```python
from build123d import *

# Parameters (mm, degrees)
SKETCH1_R           = 6.5
BOSS_EXTRUDE1_DEPTH = 25
EXTRUDE_THIN1_START = 0.5
SKETCH1_4_R         = 3.5
SKETCH1_4_R_2       = 3
EXTRUDE_THIN1_DEPTH = 20
BOSS_EXTRUDE2_START = 0.8
SKETCH1_5_R         = 5.5
SKETCH1_5_R_2       = 3
BOSS_EXTRUDE2_DEPTH = 19.5
BOSS_EXTRUDE3_START = 0.3
SKETCH1_6_R         = 6.5
SKETCH1_6_R_2       = 5.5
BOSS_EXTRUDE3_DEPTH = 21
BOSS_EXTRUDE4_START = 1
BOSS_EXTRUDE4_DEPTH = 1
FILLET1_R           = 0.5


with BuildPart() as part:
    # Sketch1 → Boss-Extrude1 (new body)
    with BuildSketch(Plane(origin=(0, 0, 0), x_dir=(0, 0, -1), z_dir=(1, 0, 0))):
        Polygon((-15, -3), (-13.5, -1.5), (-13.5, 6), (-6.5, 6), (-5, 9), (5, 9), (6.5, 6), (13.5, 6), (13.5, -1.5), (15, -3), (15, -9), (5, -9), (3.5, -7.5), (-3.5, -7.5), (-5, -9), (-15, -9), align=None)
        Circle(SKETCH1_R, mode=Mode.SUBTRACT)
    extrude(amount=BOSS_EXTRUDE1_DEPTH)



with BuildPart() as body_2:
    # Sketch1_4 → Extrude-Thin1 (new body)
    with BuildSketch(Plane(origin=(0, 0, 0), x_dir=(0, 0, -1), z_dir=(1, 0, 0)).offset(EXTRUDE_THIN1_START)):
        Circle(SKETCH1_4_R)
        Circle(SKETCH1_4_R_2, mode=Mode.SUBTRACT)
    extrude(amount=EXTRUDE_THIN1_DEPTH)

    # Sketch1_5 → Boss-Extrude2 (add)
    with BuildSketch(Plane(origin=(0, 0, 0), x_dir=(0, 0, -1), z_dir=(1, 0, 0)).offset(BOSS_EXTRUDE2_START)):
        Circle(SKETCH1_5_R)
        Circle(SKETCH1_5_R_2, mode=Mode.SUBTRACT)
    extrude(amount=BOSS_EXTRUDE2_DEPTH)


with BuildPart() as part_1:
    add(part.part)

    add(body_2.part)  # Boss-Extrude3 merges body 2
    # Sketch1_6 → Boss-Extrude3 (add)
    with BuildSketch(Plane(origin=(0, 0, 0), x_dir=(0, 0, -1), z_dir=(1, 0, 0)).offset(BOSS_EXTRUDE3_START)):
        Circle(SKETCH1_6_R)
        with Locations(Location((0, 0, 0), (0, 0, 180))):
            Circle(SKETCH1_6_R_2, mode=Mode.SUBTRACT)
    extrude(amount=BOSS_EXTRUDE3_DEPTH)

    # Sketch3 → Boss-Extrude4 (add)
    with BuildSketch(Plane(origin=(21.3, 0, 0), x_dir=(0, 0, -1), z_dir=(1, 0, 0)).offset(BOSS_EXTRUDE4_START)):
        with BuildLine():
            Line((-1.039258499, -5.400920456), (-1.22821459, -6.382905993))
            ThreePointArc((-1.22821459, -6.382905993), (0, 6.5), (1.22821459, -6.382905993))
            Line((1.22821459, -6.382905993), (1.039258499, -5.400920456))
            ThreePointArc((1.039258499, -5.400920456), (1.377808725, -4.340610122), (2.487175706, -4.250171409))
            ThreePointArc((2.487175706, -4.250171409), (3.080776399, -4.371188169), (3.635318393, -4.12728242))
            ThreePointArc((3.635318393, -4.12728242), (0, 5.5), (-3.635318393, -4.12728242))
            ThreePointArc((-3.635318393, -4.12728242), (-3.080776399, -4.371188169), (-2.487175706, -4.250171409))
            ThreePointArc((-2.487175706, -4.250171409), (-1.377808725, -4.340610122), (-1.039258499, -5.400920456))
        make_face()
    extrude(amount=BOSS_EXTRUDE4_DEPTH)

    # Fillet1
    fillet1_edges = [part_1.edges().sort_by_distance(p)[0] for p in [
        (25, -2.25, 14.25),
        (25, -6, 15),
        (0, 2.25, 13.5),
        (0, 6, 10),
        (0, 7.5, 5.75),
        (0, 9, 0),
        (0, 7.5, -5.75),
        (0, 6, -10),
        (0, 2.25, -13.5),
        (0, -2.25, -14.25),
        (0, -6, -15),
        (0, -6, 15),
        (0, -2.25, 14.25),
        (12.5, -1.5, 13.5),
        (12.5, 6, 13.5),
        (12.5, 6, 6.5),
        (12.5, 9, 5),
        (12.5, 9, -5),
        (12.5, 6, -6.5),
        (12.5, 6, -13.5),
        (12.5, -1.5, -13.5),
        (12.5, -3, -15),
        (12.5, -3, 15),
        (25, -6, -15),
        (25, -2.25, -14.25),
        (25, 2.25, -13.5),
        (25, 6, -10),
        (25, 7.5, -5.75),
        (25, 9, 0),
        (25, 7.5, 5.75),
        (25, 6, 10),
        (25, 2.25, 13.5),
    ]]
    fillet(fillet1_edges, radius=FILLET1_R)


solid = part_1.part
```
Input: part model. Units: mm. Frame: model coordinates. A direction names the side the tool comes from. Round coordinates to 2 decimals unless told otherwise and drop trailing zeros. Order: outer loops, then holes, each group sorted by start corner. A loop starts at its lowest first (then second) coordinate and runs counter-clockwise, first axis right, second up. Notation, with made-up numbers: (64, 62) - (119, 62) arc R10 ccw to (119, 79) - close; hole circle Ø3 at (-29, 62). An arc over 180 degrees is marked (long way). One line per question, with ' | ' between items. Start each with the question number.
1) Set-up query: faces 1 (the flat face through (12, -7.5, 0)), 2 (the flat face through (12, 2, 13.5)), 3 (the cylindrical face through (0.55, 5.37, -1.19)), 4 (the flat face through (20.5, 1, -3)). Return all of +Z, -Z, +X, -X, +Y, -Y with unobstructed straight access to the full face (end or side cutting, diameter ignored); none if empty.
2) Contact query for flat-ended pins moving along their axis: P1, Ø3, axis at x = 22.5, z = 11.5, coming from the +Y side; P2, Ø5, axis at x = 18, z = 9, coming from the +Y side; P3, Ø3.5, axis at y = -1, z = 1, coming from the +X side. Output: stop coordinate, or through.
3) Ray query, probe 1 along Y at (x, z) = (20.65, 0); probe 2 along Z at (x, y) = (22.75, 0); probe 3 along Y at (x, z) = (21.5, -9.5). Return the intervals inside material, ascending.
4) Cut plane B-B, the plane z = 11. Return the cut outline in (x, y), then the cut area to 3 significant figures.
5) Cut plane A-A, the plane x = 4.25. Return the cut outline in (y, z).
6) Pull-direction query (X, two-part tool) for faces 5 (the cylindrical face through (10, 0, 3)), 6 (the flat face through (22.3, -4.7, 1.4)), 7 (the cylindrical face through (24.857, -2.365, -14.152)); classes: +X half, -X half, draft (parallel to the pull), parting line (faces both ways), or undercut.
Worked out:
1) face 1: +X, -X, -Y | face 2: +Z, +X, -X, +Y | face 3: -X | face 4: +X
2) P1: stops at y = 6 | P2: stops at y = 6.11 | P3: stops at x = 20.5
3) probe 1: y = -7.5 to -5.5, 5.5 to 9 | probe 2: z = -13.5 to -5.5, 5.5 to 13.5 | probe 3: y = -9 to 6
4) outline: (0, -9) - (25, -9) - (25, 5.5) arc R0.5 ccw to (24.5, 6) - (0.5, 6) arc R0.5 ccw to (0, 5.5) - close | area: 375 mm^2
5) outline: (-9, -15) - (-3.21, -15) arc R0.5 ccw to (-2.85, -14.85) - (-1.65, -13.65) arc R0.5 cw to (-1.29, -13.5) - (5.5, -13.5) arc R0.5 ccw to (6, -13) - (6, -6.81) arc R0.5 cw to (6.28, -6.36) - (8.72, -5.14) arc R0.5 ccw to (9, -4.69) - (9, 4.69) arc R0.5 ccw to (8.72, 5.14) - (6.28, 6.36) arc R0.5 cw to (6, 6.81) - (6, 13) arc R0.5 ccw to (5.5, 13.5) - (-1.29, 13.5) arc R0.5 cw to (-1.65, 13.65) - (-2.85, 14.85) arc R0.5 ccw to (-3.21, 15) - (-9, 15) - (-9, 5) - (-7.5, 3.5) - (-7.5, -3.5) - (-9, -5) - close; hole circle Ø6 at (0, 0)
6) face 5: draft | face 6: undercut | face 7: +X half
